The model under review builds one solid part; all positions refer to its coordinate system, in mm. A direction names the side the tool comes from. Round coordinates to 2 decimals unless told otherwise and drop trailing zeros. Loops run counter-clockwise (first coordinate to the right, second up) from the corner with the lowest first, then second, coordinate; pieces in that order, holes last. Notation, with made-up numbers: M 56.5,40.5 L 97.5,40.5 A26 cw 97.5,68.5 Z; hole C -1,15 d8. An arc over 180 degrees is marked long. Answer as a JSON object with one key per item and string values. Group by question number.
Item 1: Consider section A-A (x = 0). Give the boundary of the cut face in (y, z), and give its area (3 significant figures).
Item 2: Tool access review of faces 5 (the face through (-1.497, 7.472, -0.621)), 6 (the face through (-2, -7.4, 3)): name each direction out of +Z, -Z, +X, -X, +Y, -Y from which nothing blocks a thin tool from reaching the whole face with its end or side.
Item 3: Consider section C-C (z = 0). Give the boundary of the cut face in (x, y), and give its area (3 significant figures).
Item 4: To check wall thickness, follow line 1 (X direction, y = 0, z = 2.25); line 2 (Z direction, x = 8, y = 0); line 3 (X direction, y = 2.5, z = 1.75). State the ranges of each line that lie inside material, in increasing order.
Item 5: The part is to be moulded in two halves that separate along Y. For faces 1 (the face through (3, 6, -3)), 2 (the face through (7.472, 1.497, -0.621)), 3 (the face through (-1.301, -5.857, 0.796)), 4 (the face through (-7.54, 5.78, -0.04)), say which applies: +Y half, -Y half, draft (parallel to the pull), parting line (faces both ways), or undercut.
Item 6: Insertion check: P1, Ø3, axis at x = 0, z = 0, coming from the +Y side; P2, Ø9.5, axis at x = 0, y = 0, coming from the +Z side; P3, Ø1.5, axis at y = -7.5, z = -1.5, coming from the -X side. Each pin has a flat end and moves straight along its axis. Give the tip position at first contact, or say it passes through.
Autodesk Inventor part; units mm, degrees
ref_plane "body_set_h_XY" through (0, 9.5, 0) normal (0, 1, 0) x (1, 0, 0)
ref_plane "body_set_h_YZ" through (0, 9.5, 0) normal (1, 0, 0) x (0, 0, -1)
ref_plane "body_set_h_ZX" through (0, 9.5, 0) normal (0, 0, -1) x (0, 1, 0)
sketch "Sketch_1" plane through (0, 0, 0) normal (0, 1, 0) x (-1, 0, 0)
  line L0 (0, 4.5) -> (0, -3)
  line L1 (-6, 4) -> (-6.5, 4.5)
  line L2 (-6.5, 4.5) -> (-7, 4.5)
  line L3 (-7, 4.5) -> (-7.5, 4)
  line L4 (-7.5, 4) -> (-7.5, 3)
  line L5 (-7.5, 3) -> (-9, 3)
  line L6 (-9, 3) -> (-9.5, 2.5)
  line L7 (-9.5, 2.5) -> (-9.5, -2.5)
  line L8 (-9.5, -2.5) -> (-9, -3)
  line L9 (-9, -3) -> (-6.5, -3)
  line L10 (-6.5, -3) -> (-6, -2.5)
  line L11 (-6, -2.5) -> (-6, 4)
revolve "Revolution1" add sketch "Sketch_1" angle 360 about axis through (0, 0, 4.5) along (0, 0, -1)
sketch "Sketch_8" plane through (0, 0, 0) normal (0, 0, 1) x (1, 0, 0)
  line L0 (9.5, 0) -> (5, 0)
  line L1 (5, 0) -> (5, 1.621)
  line L2 (5, 1.621) -> (9.121, 1.621)
  line L3 (9.121, 1.621) -> (9.5, 2)
  line L4 (9.5, 2) -> (9.5, 0)
  line L5 (9.5, 0) -> (5, 0)
revolve "Revolution2" cut sketch "Sketch_8" angle 360 about axis through (9.5, 0, 0) along (-1, 0, 0)
thread "Thread1"
sketch "Sketch_2" plane through (0, 0, 0) normal (0, 0, 1) x (1, 0, 0)
  line L0 (0, 9.5) -> (0, 5)
  line L1 (0, 5) -> (-1.621, 5)
  line L2 (-1.621, 5) -> (-1.621, 9.121)
  line L3 (-1.621, 9.121) -> (-2, 9.5)
  line L4 (-2, 9.5) -> (0, 9.5)
  line L5 (0, 9.5) -> (0, 5)
revolve "Revolution3" cut sketch "Sketch_2" angle 360 about axis through (0, 9.5, 0) along (0, -1, 0)
thread "Thread2"
ref_plane "body_set_h_XY" through (0, 9.5, 0) normal (0, 1, 0) x (1, 0, 0)
ref_plane "body_set_h_YZ" through (0, 9.5, 0) normal (1, 0, 0) x (0, 0, -1)
ref_plane "body_set_h_ZX" through (0, 9.5, 0) normal (0, 0, -1) x (0, 1, 0)
ref_plane "body_set_v_XY" through (9.5, 0, 0) normal (1, 0, 0) x (0, 0, -1)
ref_plane "body_set_v_YZ" through (9.5, 0, 0) normal (0, 0, -1) x (0, 1, 0)
ref_plane "body_set_v_ZX" through (9.5, 0, 0) normal (0, 1, 0) x (1, 0, 0)
properties part number "SCBRJ12-15_b"
Geometry results:
{
 "1": {"outline": "M -9.5,-2.5 L -9,-3 L -6.5,-3 L -6,-2.5 L -6,4 L -6.5,4.5 L -7,4.5 L -7.5,4 L -7.5,3 L -9,3 L -9.5,2.5 Z; M 6,-2.5 L 6.5,-3 L 9,-3 L 9.5,-2.5 L 9.5,-2 L 9.12,-1.62 L 6,-1.62 Z; M 6,1.62 L 9.12,1.62 L 9.5,2 L 9.5,2.5 L 9,3 L 7.5,3 L 7.5,4 L 7,4.5 L 6.5,4.5 L 6,4 Z", "area": "33.8 mm^2"},
 "2": {"face 5": "+Y", "face 6": "+Z"},
 "3": {"outline": "M -1.82,9.32 A9.5 ccw long 9.32,-1.82 L 9.12,-1.62 L 5.78,-1.62 A6 cw long -1.62,5.78 L -1.62,9.12 Z; M 1.62,5.78 A6 cw 5.78,1.62 L 9.12,1.62 L 9.32,1.82 A9.5 ccw 1.82,9.32 L 1.62,9.12 Z", "area": "147 mm^2"},
 "4": {"line 1": "x = -9.5 to -6, 6 to 9.5", "line 2": "z = -3 to -1.62, 1.62 to 3", "line 3": "x = -9.17 to -5.45, 5.45 to 9.17"},
 "5": {"face 1": "draft", "face 2": "undercut", "face 3": "undercut", "face 4": "parting line"},
 "6": {"P1": "stops at y = -5.81", "P2": "passes through", "P3": "stops at x = -6.68"}
}
